```python
from build123d import *

# Parameters (mm, degrees)
F1_DEPTH = 1.905
F2_DEPTH = 1.905


with BuildPart() as f1:
    # F0 (on Front) → F1 (new body)
    with BuildSketch(Plane.XZ):
        Polygon((-275.385344, 43.545973), (-275.385344, -210.454027), (258.014656, -210.454027), (258.014656, 43.545973), (67.514656, 43.545973), (67.514656, 221.345973), (-84.885344, 221.345973), (-84.885344, 43.545973), align=None)
        Polygon((-82.980344, 219.440973), (65.609656, 219.440973), (65.609656, 41.640973), (256.109656, 41.640973), (256.109656, -208.549027), (-273.480344, -208.549027), (-273.480344, 41.640973), (-82.980344, 41.640973), align=None, mode=Mode.SUBTRACT)
    extrude(amount=F1_DEPTH)

    # F0 (on Front) → F2 (join)
    with BuildSketch(Plane.XZ):
        Polygon((-275.385344, 43.545973), (-275.385344, -210.454027), (258.014656, -210.454027), (258.014656, 43.545973), (67.514656, 43.545973), (67.514656, 221.345973), (-84.885344, 221.345973), (-84.885344, 43.545973), align=None)
        Polygon((-82.980344, 219.440973), (65.609656, 219.440973), (65.609656, 41.640973), (256.109656, 41.640973), (256.109656, -208.549027), (-273.480344, -208.549027), (-273.480344, 41.640973), (-82.980344, 41.640973), align=None, mode=Mode.SUBTRACT)
        Polygon((65.609656, 41.640973), (65.609656, 219.440973), (-82.980344, 219.440973), (-82.980344, 41.640973), (-273.480344, 41.640973), (-273.480344, -208.549027), (256.109656, -208.549027), (256.109656, 41.640973), align=None)
    extrude(amount=F2_DEPTH)


solid = f1.part
```
Check sheet for the modelled part. Datum: model origin and axes. Units: mm. Round coordinates to 2 decimals unless told otherwise and drop trailing zeros. Write each loop counter-clockwise with the first axis right and the second up, starting at its lowest first coordinate (ties: lowest second). Pieces come first, ordered by that corner, then holes. Notation, with made-up numbers: (-13, 9.5) -> (5, 9.5) arc R19 ccw to (5, 39.5) -> close; hole circle Ø5 at (89.5, -23). An arc over 180 degrees is marked (long way). Put each result on its own line as item: value.
(1) Sectioned sample at B-B (z = 128). Enter the section's corners in (x, y) (3 decimals).
Values found:
outline: (-84.885, -1.905) -> (67.515, -1.905) -> (67.515, 0) -> (-84.885, 0) -> close
(2) Material ranges on line 1 (Z direction, x = 195.5, y = -0.85); line 2 (X direction, y = -0.35, z = 107), recorded low to high.
Values found:
line 1: z = -210.45 to 43.55
line 2: x = -84.89 to 67.51
(3) Sectioned sample at C-C (x = 202.5). Enter the section's corners in (y, z) (3 decimals).
Values found:
outline: (-1.905, -210.454) -> (0, -210.454) -> (0, 43.546) -> (-1.905, 43.546) -> close
(4) Go/stop test with flat-tipped pins: pin 1 Ø1 at (y, z) = (-1, 103) entering from -X; pin 2 Ø1 at (x, y) = (84.5, -1.5) entering from +Z. Record where each tip stops, or that it passes through.
Values found:
pin 1: stops at x = -84.89
pin 2: stops at z = 43.55
(5) Sectioned sample at A-A (y = -1.4). Enter the section's corners in (x, z).
Values found:
outline: (-275.39, -210.45) -> (258.01, -210.45) -> (258.01, 43.55) -> (67.51, 43.55) -> (67.51, 221.35) -> (-84.89, 221.35) -> (-84.89, 43.55) -> (-275.39, 43.55) -> close
